Read the model definition and answer for the solid it produces. Units are mm, in the model's axes. A direction names the side the tool comes from. Give positions to 0.01 mm unless a question says otherwise; leave off trailing zeros. Write each loop counter-clockwise with the first axis right and the second up, starting at its lowest first coordinate (ties: lowest second). Pieces come first, ordered by that corner, then holes. Notation, with made-up numbers: M 42.25,50 L 96.25,50 A13 cw 96.25,59 Z; hole C 56,89 d10. An arc over 180 degrees is marked long. Put each result on its own line as item: value.
from build123d import *

# Parameters (mm, degrees)
SKETCH3_W           = 304.898736347
SKETCH3_H           = 152.426093062
BOSS_EXTRUDE1_DEPTH = 101.6
SKETCH4_W           = 63.5
SKETCH4_H           = 50.8
CUT_EXTRUDE1_DEPTH  = 147.32
SKETCH5_W           = 254.098736347
SKETCH5_H           = 101.626093062
SKETCH5_R           = 19.05
CUT_EXTRUDE2_DEPTH  = 76.2
CUT_EXTRUDE3_START  = 138.938
SKETCH7_R           = 19.05
CUT_EXTRUDE3_DEPTH  = 138.938


with BuildPart() as part:
    # Sketch3 → Boss-Extrude1 (new body)
    with BuildSketch(Plane(origin=(0, 0, 0), x_dir=(1, 0, 0), z_dir=(0, 1, 0))):
        with Locations((152.449368174, 76.213046531)):
            Rectangle(SKETCH3_W, SKETCH3_H)
    extrude(amount=BOSS_EXTRUDE1_DEPTH)

    # Sketch4 → Cut-Extrude1 (cut)
    with BuildSketch(Plane(origin=(0, 0, 0), x_dir=(1, 0, 0), z_dir=(0, 1, 0))):
        with Locations((273.148736347, 76.226093062)):
            Rectangle(SKETCH4_W, SKETCH4_H)
    extrude(amount=CUT_EXTRUDE1_DEPTH, mode=Mode.SUBTRACT)

    # Sketch5 → Cut-Extrude2 (cut)
    with BuildSketch(Plane(origin=(0, 101.6, 0), x_dir=(1, 0, 0), z_dir=(0, 1, 0))):
        with Locations((152.449368174, 76.213046531)):
            Rectangle(SKETCH5_W, SKETCH5_H)
        with Locations(Location((76.2, 76.226093062, 0), (0, 0, 270))):
            Circle(SKETCH5_R, mode=Mode.SUBTRACT)
        with Locations(Location((133.35, 76.226093062, 0), (0, 0, 270))):
            Circle(SKETCH5_R, mode=Mode.SUBTRACT)
        with Locations(Location((190.5, 76.226093062, 0), (0, 0, 270))):
            Circle(SKETCH5_R, mode=Mode.SUBTRACT)
    extrude(amount=-CUT_EXTRUDE2_DEPTH, mode=Mode.SUBTRACT)

    # Sketch7 → Cut-Extrude3 (cut)
    with BuildSketch(Plane(origin=(0, 0, 0), x_dir=(1, 0, 0), z_dir=(0, 1, 0)).offset(CUT_EXTRUDE3_START)):
        with Locations(Location((76.2, 76.226093062, 0), (0, 0, 270))):
            Circle(SKETCH7_R)
        with Locations(Location((133.35, 76.226093062, 0), (0, 0, 270))):
            Circle(SKETCH7_R)
        with Locations(Location((190.5, 76.226093062, 0), (0, 0, 270))):
            Circle(SKETCH7_R)
    extrude(amount=-CUT_EXTRUDE3_DEPTH, mode=Mode.SUBTRACT)


solid = part.part
(1) Section D-D on y = 85.5 is taken. Determine the outline of the cut face in (x, z).
Result:
outline: M 0,-152.43 L 304.9,-152.43 L 304.9,-101.63 L 279.5,-101.63 L 279.5,-127.03 L 25.4,-127.03 L 25.4,-25.4 L 279.5,-25.4 L 279.5,-50.83 L 304.9,-50.83 L 304.9,0 L 0,0 Z
(2) Which of the six approach directions +Z, -Z, +X, -X, +Y, -Y give full straight-line access (tool end or side, diameter ignored) to faces 1 (the face through (150, 101.6, -128)), 2 (the face through (25.4, 64, -76)), 3 (the face through (287, 39, -101.626))?
Result:
face 1: +Z, -Z, +X, -X, +Y
face 2: +Y
face 3: +X, +Y, -Y
(3) Straight lines are drawn through the part: line 1 along Z through (x, y) = (25.5, 87.5); line 2 along X through (y, z) = (14.5, -66); line 3 along X through (y, z) = (86, -26). For each, find the intervals that lie inside material, in ascending order. Write a range as from..to.
Result:
line 1: z = -152.43..-127.03, -25.4..0
line 2: x = 0..60.13, 92.27..117.28, 149.42..174.43, 206.57..241.4
line 3: x = 0..25.4, 279.5..304.9
(4) Given pin 1 Ø7.5 at (y, z) = (10, -67) entering from +X; pin 2 Ø5 at (x, z) = (65.5, -52.5) entering from +Y, each flat-ended and moving along its own axis, determine where each tip first touches the part or whether it passes through.
Result:
pin 1: stops at x = 241.4
pin 2: stops at y = 25.4
(5) For a pull along X with two mould halves and no side action, classify faces 4 (the face through (150, 50, 0)), 5 (the face through (279.499, 64, -38)), 6 (the face through (241.399, 13, -76)) as +X half, -X half, draft (parallel to the pull), parting line (faces both ways), or undercut.
Result:
face 4: draft
face 5: undercut
face 6: +X half
(6) Section A-A on x = 133.35 is taken. Determine the outline of the cut face in (y, z), and give its area (3 significant figures).
Result:
outline: M 0,-152.43 L 101.6,-152.43 L 101.6,-127.03 L 25.4,-127.03 L 25.4,-95.28 L 0,-95.28 Z; M 0,-57.18 L 25.4,-57.18 L 25.4,-25.4 L 101.6,-25.4 L 101.6,0 L 0,0 Z
area: 6,770 mm²
(7) Section B-B on z = -65 is taken. Determine the outline of the cut face in (x, y).
Result:
outline: M 0,0 L 60.81,0 L 60.81,25.4 L 25.4,25.4 L 25.4,101.6 L 0,101.6 Z; M 91.59,0 L 117.96,0 L 117.96,25.4 L 91.59,25.4 Z; M 148.74,0 L 175.11,0 L 175.11,25.4 L 148.74,25.4 Z; M 205.89,0 L 241.4,0 L 241.4,25.4 L 205.89,25.4 Z
(8) Section C-C on y = 17 is taken. Determine the outline of the cut face in (x, z).
Result:
outline: M 0,-152.43 L 304.9,-152.43 L 304.9,-101.63 L 241.4,-101.63 L 241.4,-50.83 L 304.9,-50.83 L 304.9,0 L 0,0 Z; hole C 76.2,-76.23 d38.1; hole C 133.35,-76.23 d38.1; hole C 190.5,-76.23 d38.1
